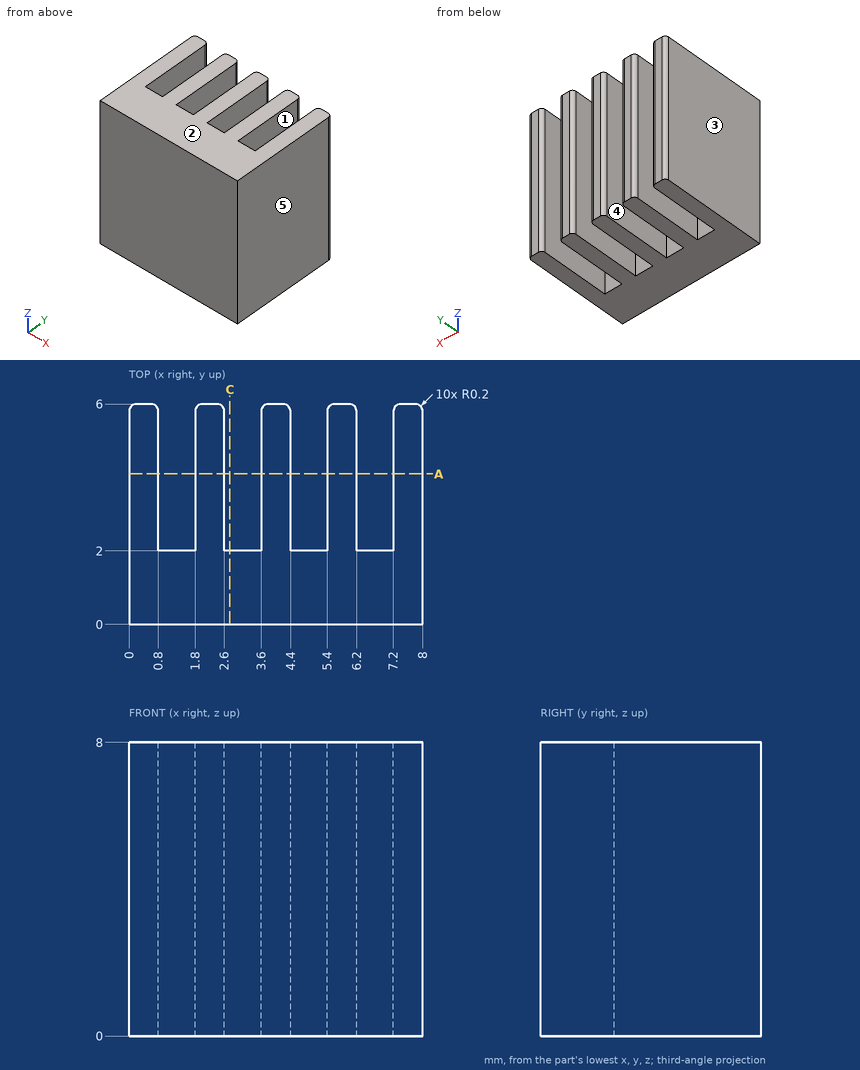
Design review of the part shown in the three views and the two pictorial views. Dimensions are in mm from the part's minimum x, y and z. A direction names the side the tool comes from. Round coordinates to 2 decimals unless told otherwise and drop trailing zeros. Write each loop counter-clockwise with the first axis right and the second up, starting at its lowest first coordinate (ties: lowest second). Pieces come first, ordered by that corner, then holes.
1) Take a section at C-C on x = 2.75. Give the boundary of the cut face in (y, z).
Answer below:
outline: (0, 0) - (2, 0) - (2, 8) - (0, 8) - close
2) For line 1 along X through (y, z) = (5.75, 1.5); line 2 along Y through (x, z) = (3, 7.25); line 3 along Y through (x, z) = (4.25, 6.25), list the stretches that pass through material, from the lowest coordinate up.
Answer below:
line 1: x = 0 to 0.8, 1.8 to 2.6, 3.6 to 4.4, 5.4 to 6.2, 7.2 to 8
line 2: y = 0 to 2
line 3: y = 0 to 5.99
3) Take a section at A-A on y = 4.1. Give the boundary of the cut face in (x, z), then the cut area to 3 significant figures.
Answer below:
outline: (0, 0) - (0.8, 0) - (0.8, 8) - (0, 8) - close; (1.8, 0) - (2.6, 0) - (2.6, 8) - (1.8, 8) - close; (3.6, 0) - (4.4, 0) - (4.4, 8) - (3.6, 8) - close; (5.4, 0) - (6.2, 0) - (6.2, 8) - (5.4, 8) - close; (7.2, 0) - (8, 0) - (8, 8) - (7.2, 8) - close
area: 32.0 mm2
4) Mouldability with a two-part tool opening along X and no side actions: class the marked faces 1, 2 and 3 as +X half, -X half, draft (parallel to the pull), parting line (faces both ways), or undercut.
Answer below:
face 1: undercut
face 2: draft
face 3: -X half
5) Machinability: for the marked faces 4 and 5, which of the approach directions +Z, -Z, +X, -X, +Y, -Y give a long, thin tool a straight path to every point of the face, cutting with its end or side? Answer none if there is none.
Answer below:
face 4: +Z, -Z, +Y
face 5: +Z, -Z, +X, +Y, -Y
6) Insertion check: pin 1 Ø0.5 at (x, z) = (6.5, 2) entering from +Y; pin 2 Ø1.1 at (x, z) = (3, 5) entering from +Y. Each pin has a flat end and moves straight along its axis. Give the tip position at first contact, or say it passes through.
Answer below:
pin 1: stops at y = 2
pin 2: stops at y = 5.99
